Design review of the part built by this model. Coordinates are the model's own, in mm. A direction names the side the tool comes from. Give positions to 0.01 mm unless a question says otherwise; leave off trailing zeros. Loops run counter-clockwise (first coordinate to the right, second up) from the corner with the lowest first, then second, coordinate; pieces in that order, holes last. Notation, with made-up numbers: M 76.5,32.25 L 99.5,32.25 A33 ccw 99.5,66.25 Z; hole C 5.5,-12.5 d6. An arc over 180 degrees is marked long. Use a Markdown table: item, result. Add a question column.
(1) Add section A-A, the plane y = 48.5. Give the boundary of the cut face in (x, z).
(2) Add section D-D, the plane z = 44. Give the boundary of the cut face in (x, y).
(3) For faces 1 (the face through (181, 92.052, 105)), 2 (the face through (39, 6, 98)), 3 (the face through (56, 11, 32.703)), 4 (the face through (5, 90, 159.195)), list the 3-axis set-ups (+Z, -Z, +X, -X, +Y, -Y) from which the entire face can be reached by the end or side of a thin tool; tool diameter is ignored.
(4) Insertion check: pin 1 Ø10 at (x, y) = (52, 16) entering from -Z; pin 2 Ø1.8 at (x, z) = (39, 120) entering from +Y; pin 3 Ø2 at (x, z) = (68, 34.5) entering from +Y. Each pin has a flat end and moves straight along its axis. Give the tip position at first contact, or say it passes through.
(5) Add section B-B, the plane y = 82. Give the boundary of the cut face in (x, z), then the cut area to 3 significant figures.
(6) For probe 1 along X at (y, z) = (113, 7); probe 2 along X at (y, z) = (14, 114); probe 3 along X at (y, z) = (46.5, 144), list the stretches that pass through material, from the lowest coordinate up.
(7) Draft analysis for pull direction X (two halves, no side actions). For faces 5 (the face through (147, 6, 98)), 6 (the face through (186, 59, 82)), 7 (the face through (5, 87.052, 105)), state which applies: pulls with the +X half, pulls with the -X half, needs draft (parallel to the pull), parting line crosses it, or undercut.
(8) Add section C-C, the plane z = 151. Give the boundary of the cut face in (x, y).
```python
from build123d import *

# Parameters (mm, degrees)
EXTRUDE_THIN2_DEPTH     = 165.4
SKETCH11_W              = 163
SKETCH11_H              = 4
BOSS_EXTRUDE3_DEPTH     = 2.6416
CUT_EXTRUDE6_DEPTH      = 270.69086006
CUT_EXTRUDE6_DEPTH_BACK = 270.69086006
SKETCH13_W              = 110.495011338
SKETCH13_H              = 5
CUT_EXTRUDE7_DEPTH      = 273.127102656
SKETCH19_W              = 4
SKETCH19_H              = 155.4
CUT_EXTRUDE9_DEPTH      = 10
SKETCH20_W              = 4
SKETCH20_H              = 155.4
CUT_EXTRUDE10_DEPTH     = 10
SKETCH21_W              = 6
SKETCH21_H              = 86.697
BOSS_EXTRUDE4_DEPTH     = 110
CUT_EXTRUDE11_DEPTH     = 4
SKETCH23_W              = 163
SKETCH23_H              = 4
BOSS_EXTRUDE5_DEPTH     = 2.6416
SKETCH24_W              = 2.6416
SKETCH24_H              = 4
BOSS_EXTRUDE6_DEPTH     = 49.6416
SKETCH25_W              = 2.64
SKETCH25_H              = 4
BOSS_EXTRUDE7_DEPTH     = 49.6416
SKETCH26_W              = 2.64
SKETCH26_H              = 4
BOSS_EXTRUDE8_DEPTH     = 49.6416


with BuildPart() as part:
    # Sketch2 → Extrude-Thin2 (new body)
    with BuildSketch(Plane.XY):
        Polygon((0, 120), (0, 0), (186, 0), (186, 120), (176, 120), (176, 10), (10, 10), (10, 120), align=None)
    extrude(amount=EXTRUDE_THIN2_DEPTH)

    # Sketch11 → Boss-Extrude3 (add)
    with BuildSketch(Plane(origin=(0, 10, 0), x_dir=(1, 0, 0), z_dir=(0, 1, 0))):
        with Locations((93, -34.703)):
            Rectangle(SKETCH11_W, SKETCH11_H)
    extrude(amount=BOSS_EXTRUDE3_DEPTH)

    # Sketch13 → Cut-Extrude6 (cut, two sides: drawn at the far end of the back side and taken through both)
    with BuildSketch(Plane(origin=(10, 0, 0), x_dir=(0, 0, -1), z_dir=(1, 0, 0)).offset(-CUT_EXTRUDE6_DEPTH_BACK)):
        with Locations((-103.947505669, 89.551599899)):
            Rectangle(SKETCH13_W, SKETCH13_H)
    extrude(amount=CUT_EXTRUDE6_DEPTH + CUT_EXTRUDE6_DEPTH_BACK, mode=Mode.SUBTRACT)

    # Sketch14 → Cut-Extrude7 (cut, through all)
    with BuildSketch(Plane(origin=(0, 10, 0), x_dir=(1, 0, 0), z_dir=(0, 1, 0))):
        with BuildLine():
            Line((176, -165.4), (10, -165.4))
            ThreePointArc((10, -165.4), (93, -135.4), (176, -165.4))
        make_face()
    extrude(amount=-CUT_EXTRUDE7_DEPTH, mode=Mode.SUBTRACT)

    # Sketch19 → Cut-Extrude9 (cut)
    with BuildSketch(Plane(origin=(0, 120, 0), x_dir=(1, 0, 0), z_dir=(0, 1, 0))):
        with Locations((5, -82.7)):
            Rectangle(SKETCH19_W, SKETCH19_H)
    extrude(amount=-CUT_EXTRUDE9_DEPTH, mode=Mode.SUBTRACT)

    # Sketch20 → Cut-Extrude10 (cut)
    with BuildSketch(Plane(origin=(0, 120, 0), x_dir=(1, 0, 0), z_dir=(0, 1, 0))):
        with Locations((181, -82.7)):
            Rectangle(SKETCH20_W, SKETCH20_H)
    extrude(amount=-CUT_EXTRUDE10_DEPTH, mode=Mode.SUBTRACT)

    # Sketch21 → Boss-Extrude4 (add, through all)
    with BuildSketch(Plane(origin=(0, 10, 0), x_dir=(1, 0, 0), z_dir=(0, 1, 0))):
        with Locations((93, -82.0515)):
            Rectangle(SKETCH21_W, SKETCH21_H)
    extrude(amount=BOSS_EXTRUDE4_DEPTH)

    # Sketch22 → Cut-Extrude11 (cut)
    with BuildSketch(Plane(origin=(0, 10, 0), x_dir=(1, 0, 0), z_dir=(0, 1, 0))):
        Polygon((36, -48.703), (36, -148.583194008), (42, -145.837577441), (42, -48.703), align=None)
        Polygon((144, -145.837577441), (150, -148.583194008), (150, -48.703), (144, -48.703), align=None)
    extrude(amount=-CUT_EXTRUDE11_DEPTH, mode=Mode.SUBTRACT)

    # Sketch23 → Boss-Extrude5 (add)
    with BuildSketch(Plane(origin=(0, 10, 0), x_dir=(1, 0, 0), z_dir=(0, 1, 0))):
        with Locations((93, -27.4)):
            Rectangle(SKETCH23_W, SKETCH23_H)
    extrude(amount=BOSS_EXTRUDE5_DEPTH)

    # Sketch24 → Boss-Extrude6 (add)
    with BuildSketch(Plane(origin=(0, 12.6416, 0), x_dir=(1, 0, 0), z_dir=(0, 1, 0))):
        with Locations((12.8208, -34.703)):
            Rectangle(SKETCH24_W, SKETCH24_H)
    extrude(amount=BOSS_EXTRUDE6_DEPTH)

    # Sketch25 → Boss-Extrude7 (add)
    with BuildSketch(Plane(origin=(0, 12.6416, 0), x_dir=(1, 0, 0), z_dir=(0, 1, 0))):
        with Locations((12.82, -27.4)):
            Rectangle(SKETCH25_W, SKETCH25_H)
    extrude(amount=BOSS_EXTRUDE7_DEPTH)

    # Sketch26 → Boss-Extrude8 (add)
    with BuildSketch(Plane(origin=(0, 12.6416, 0), x_dir=(1, 0, 0), z_dir=(0, 1, 0))):
        with Locations((173.18, -34.703)):
            Rectangle(SKETCH26_W, SKETCH26_H)
        with Locations((173.18, -27.4)):
            Rectangle(SKETCH26_W, SKETCH26_H)
    extrude(amount=BOSS_EXTRUDE8_DEPTH)


solid = part.part
```
Established:
| question | item | result |
|---|---|---|
| 1 | outline | M 0,0 L 10,0 L 10,165.4 L 0,165.4 Z; M 11.5,25.4 L 14.14,25.4 L 14.14,29.4 L 11.5,29.4 Z; M 11.5,32.7 L 14.14,32.7 L 14.14,36.7 L 11.5,36.7 Z; M 90,38.7 L 96,38.7 L 96,125.4 L 90,125.4 Z; M 171.86,25.4 L 174.5,25.4 L 174.5,29.4 L 171.86,29.4 Z; M 171.86,32.7 L 174.5,32.7 L 174.5,36.7 L 171.86,36.7 Z; M 176,0 L 186,0 L 186,165.4 L 176,165.4 Z |
| 2 | outline | M 0,0 L 186,0 L 186,120 L 183,120 L 183,110 L 179,110 L 179,120 L 176,120 L 176,10 L 96,10 L 96,120 L 90,120 L 90,10 L 10,10 L 10,120 L 7,120 L 7,110 L 3,110 L 3,120 L 0,120 Z |
| 3 | face 1 | +X |
| 3 | face 2 | +Z, +Y |
| 3 | face 3 | +Y |
| 3 | face 4 | +X, -X |
| 4 | pin 1 | z = 25.4 |
| 4 | pin 2 | y = 6 |
| 4 | pin 3 | y = 12.64 |
| 5 | outline | M 0,0 L 10,0 L 10,165.4 L 0,165.4 Z; M 90,38.7 L 96,38.7 L 96,125.4 L 90,125.4 Z; M 176,0 L 186,0 L 186,165.4 L 176,165.4 Z |
| 5 | area | 3,830 mm^2 |
| 6 | probe 1 | 0 to 3, 7 to 10, 176 to 179, 183 to 186 |
| 6 | probe 2 | 0 to 10, 90 to 96, 176 to 186 |
| 6 | probe 3 | 0 to 10, 176 to 186 |
| 7 | face 5 | undercut |
| 7 | face 6 | pulls with the +X half |
| 7 | face 7 | needs draft |
| 8 | outline | M 0,0 L 31.3,0 L 31.3,10 L 10,10 L 10,87.05 L 0,87.05 Z; M 0,92.05 L 10,92.05 L 10,120 L 7,120 L 7,110 L 3,110 L 3,120 L 0,120 Z; M 154.7,0 L 186,0 L 186,87.05 L 176,87.05 L 176,10 L 154.7,10 Z; M 176,92.05 L 186,92.05 L 186,120 L 183,120 L 183,110 L 179,110 L 179,120 L 176,120 Z |
